Input: part model. Units: mm. Frame: model coordinates. Coordinates: 2 decimals unless noted, no trailing zeros. Loops run counter-clockwise (first coordinate to the right, second up) from the corner with the lowest first, then second, coordinate; pieces in that order, holes last.
```python
from build123d import *

# Parameters (mm, degrees)
F0_R     = 19
F0_R_2   = 6
F1_DEPTH = 10


with BuildPart() as f1:
    # F0 (on Front) → F1 (new body)
    with BuildSketch(Plane.XZ):
        with BuildLine():
            ThreePointArc((35.678131, 37.479843), (19.676649, 37.805392), (14.436751, 52.928119))
            ThreePointArc((14.436751, 52.928119), (4.2732, 71.378448), (-14.317337, 61.473684))
            Line((-14.317337, 61.473684), (-30.543653, 9.54386))
            ThreePointArc((-30.543653, 9.54386), (-30.013481, -11.099143), (-16.985078, -27.120235))
            ThreePointArc((-16.985078, -27.120235), (-11.413054, -36.106142), (-15.111724, -46.011385))
            ThreePointArc((-15.111724, -46.011385), (-20.441985, -70.131743), (0, -84))
            ThreePointArc((0, -84), (21.7408, -81.137769), (42, -72.746134))
            ThreePointArc((42, -72.746134), (52.830446, -56.419677), (46.347556, -37.931198))
            ThreePointArc((46.347556, -37.931198), (36.8637, -11.500057), (51.87381, 12.232733))
            ThreePointArc((51.87381, 12.232733), (56.625543, 33.099115), (35.678131, 37.479843))
        make_face()
        with BuildLine():
            ThreePointArc((0, -74), (-12, -62), (0, -50))
            ThreePointArc((0, -50), (12.940952, -48.296291), (25, -43.30127))
            ThreePointArc((25, -43.30127), (41.392305, -47.693575), (37, -64.08588))
            ThreePointArc((37, -64.08588), (19.152609, -71.478511), (0, -74))
        make_face(mode=Mode.SUBTRACT)
        Circle(F0_R, mode=Mode.SUBTRACT)
        with Locations((0, 57)):
            Circle(F0_R_2, mode=Mode.SUBTRACT)
        with Locations((44, 25)):
            Circle(F0_R_2, mode=Mode.SUBTRACT)
    extrude(amount=F1_DEPTH)


solid = f1.part
```
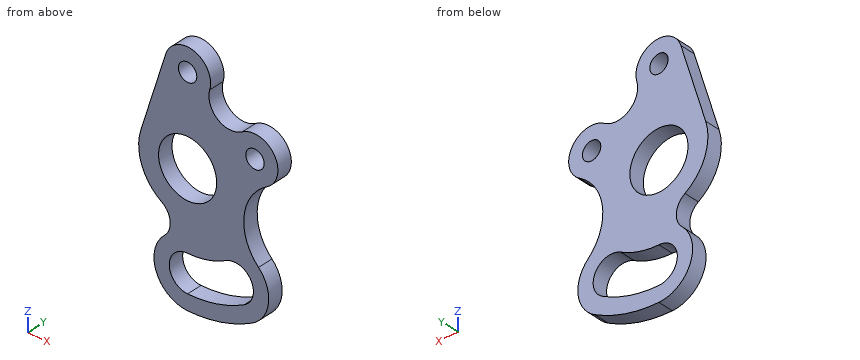
Item 1: Line query: L1, parallel to Z at x = 42, y = -7.75; L2, parallel to Z at x = -13, y = -5.5; L3, parallel to Z at x = -4, y = -8. Output: solid intervals per line, ascending.
Result:
L1: z = -72.75 to -58.49, -48.9 to -32.69, 2.68 to 19.34, 30.66 to 39.87
L2: z = -79.75 to -43.36, -31.23 to -13.86, 13.86 to 64.48
L3: z = -83.63 to -73.31, -50.69 to -18.57, 18.57 to 52.53, 61.47 to 71.46
Item 2: Section query B-B (x = 2.5). Output: boundary loops of the cut face in (y, z).
Result:
outline: (-10, -83.96) - (0, -83.96) - (0, -73.96) - (-10, -73.96) - close; (-10, -49.94) - (0, -49.94) - (0, -18.83) - (-10, -18.83) - close; (-10, 18.83) - (0, 18.83) - (0, 51.55) - (-10, 51.55) - close; (-10, 62.45) - (0, 62.45) - (0, 71.79) - (-10, 71.79) - close
Item 3: Section query A-A (z = 0). Output: boundary loops of the cut face in (x, y).
Result:
outline: (-32, -10) - (-19, -10) - (-19, 0) - (-32, 0) - close; (19, -10) - (40.41, -10) - (40.41, 0) - (19, 0) - close
Item 4: Contact query for flat-ended pins moving along their axis: P1, Ø4, axis at y = -3, z = 44.5, coming from the -X side; P2, Ø5, axis at y = -6.5, z = 50.5, coming from the -X side. Output: stop coordinate, or through.
Result:
P1: stops at x = -20.25
P2: stops at x = -18.53
Item 5: Section query C-C (y = -8.5). Output: boundary loops of the cut face in (x, z).
Result:
outline: (-30.54, 9.54) arc R32 ccw to (-16.99, -27.12) arc R12 cw to (-15.11, -46.01) arc R22 ccw to (0, -84) arc R84 ccw to (42, -72.75) arc R22 ccw to (46.35, -37.93) arc R32 cw to (51.87, 12.23) arc R15 ccw (long way) to (35.68, 37.48) arc R14 cw to (14.44, 52.93) arc R15 ccw to (-14.32, 61.47) - close; hole circle Ø38 at (0, 0); hole circle Ø12 at (0, 57); hole (0, -74) arc R74 ccw to (37, -64.09) arc R12 ccw to (25, -43.3) arc R50 cw to (0, -50) arc R12 ccw to start; hole circle Ø12 at (44, 25)
Item 6: Section query D-D (z = 25). Output: boundary loops of the cut face in (x, y).
Result:
outline: (-25.71, -10) - (38, -10) - (38, 0) - (-25.71, 0) - close; (50, -10) - (59, -10) - (59, 0) - (50, 0) - close
